Can you work these out from the model? Positions are in its coordinate system, mm. A direction names the side the tool comes from. Give positions to 0.01 mm unless a question says otherwise; leave off trailing zeros. Write each loop counter-clockwise with the first axis right and the second up, starting at its lowest first coordinate (ties: lowest second). Pieces come first, ordered by that corner, then holes.
from build123d import *

# Parameters (mm, degrees)
SKETCH1_R           = 10
BOSS_EXTRUDE1_DEPTH = 25
SKETCH2_R           = 4
CUT_EXTRUDE1_DEPTH  = 12.5
SKETCH3_R           = 2.5
CUT_EXTRUDE2_DEPTH  = 12.5
FILLET1_R           = 0.5
CHAMFER2_SIZE       = 0.5
CHAMFER3_SIZE       = 0.35
SKETCH4_R           = 3
CUT_EXTRUDE3_DEPTH  = 8
SKETCH5_R           = 1.25
CUT_EXTRUDE4_DEPTH  = 30.478806021
SKETCH6_W           = 1
SKETCH6_H           = 25
CUT_EXTRUDE5_DEPTH  = 13.95
SKETCH7_W           = 20.006481037
SKETCH7_H           = 0.5
CUT_EXTRUDE6_DEPTH  = 10.5
CUT_EXTRUDE7_START  = 13.975
SKETCH8_R           = 4
CUT_EXTRUDE7_DEPTH  = 13.975


with BuildPart() as part:
    # Sketch1 → Boss-Extrude1 (new body)
    with BuildSketch(Plane(origin=(0, 0, 0), x_dir=(1, 0, 0), z_dir=(0, 1, 0))):
        with Locations(Location((0, 0, 0), (0, 0, 270))):
            Circle(SKETCH1_R)
    extrude(amount=BOSS_EXTRUDE1_DEPTH)

    # Sketch2 → Cut-Extrude1 (cut)
    with BuildSketch(Plane(origin=(0, 25, 0), x_dir=(1, 0, 0), z_dir=(0, 1, 0))):
        with Locations(Location((0, 0, 0), (0, 0, 270))):
            Circle(SKETCH2_R)
    extrude(amount=-CUT_EXTRUDE1_DEPTH, mode=Mode.SUBTRACT)

    # Sketch3 → Cut-Extrude2 (cut)
    with BuildSketch(Plane.XZ):
        with Locations(Location((0, 0, 0), (0, 0, 270))):
            Circle(SKETCH3_R)
    extrude(amount=-CUT_EXTRUDE2_DEPTH, mode=Mode.SUBTRACT)

    # Fillet1
    fillet1_edges = [part.edges().sort_by_distance(p)[0] for p in [
        (0, 0, 2.5),
        (0, 25, -4),
    ]]
    fillet(fillet1_edges, radius=FILLET1_R)

    # Chamfer2
    chamfer2_edges = [part.edges().sort_by_distance(p)[0] for p in [
        (0, 12.5, 2.5),
    ]]
    chamfer(chamfer2_edges, length=CHAMFER2_SIZE)

    # Chamfer3
    chamfer3_edges = [part.edges().sort_by_distance(p)[0] for p in [
        (0, 0, -10),
        (0, 25, -10),
    ]]
    chamfer(chamfer3_edges, length=CHAMFER3_SIZE)

    # Sketch4 → Cut-Extrude3 (cut)
    with BuildSketch(Plane.ZY.offset(-10)):
        with Locations((-7, 19)):
            Circle(SKETCH4_R)
        with Locations((-7, 6)):
            Circle(SKETCH4_R)
    extrude(amount=CUT_EXTRUDE3_DEPTH, mode=Mode.SUBTRACT)

    # Sketch5 → Cut-Extrude4 (cut, through all)
    with BuildSketch(Plane(origin=(2, 0, 0), x_dir=(0, 0, -1), z_dir=(1, 0, 0))):
        with Locations((7, 19)):
            Circle(SKETCH5_R)
        with Locations((7, 6)):
            Circle(SKETCH5_R)
    extrude(amount=-CUT_EXTRUDE4_DEPTH, mode=Mode.SUBTRACT)

    # Sketch6 → Cut-Extrude5 (cut)
    with BuildSketch(Plane.XY.offset(-10)):
        with Locations((0, 12.5)):
            Rectangle(SKETCH6_W, SKETCH6_H)
    extrude(amount=CUT_EXTRUDE5_DEPTH, mode=Mode.SUBTRACT)

    # Sketch7 → Cut-Extrude6 (cut)
    with BuildSketch(Plane.ZY.offset(-10)):
        with Locations((0.003240519, 12.5)):
            Rectangle(SKETCH7_W, SKETCH7_H)
    extrude(amount=CUT_EXTRUDE6_DEPTH, mode=Mode.SUBTRACT)

    # Sketch8 → Cut-Extrude7 (cut)
    with BuildSketch(Plane(origin=(0, 12.25, 0), x_dir=(1, 0, 0), z_dir=(0, 1, 0)).offset(CUT_EXTRUDE7_START)):
        Circle(SKETCH8_R)
    extrude(amount=-CUT_EXTRUDE7_DEPTH, mode=Mode.SUBTRACT)


solid = part.part
(1) Imagine slicing it at D-D, the plane y = 6. Write out the boundary of the cut face in (x, z).
Returned:
outline: (-8.18, -5.75) - (-0.5, -5.75) - (-0.5, -2.45) arc R2.5 cw to (-0.5, 2.45) - (-0.5, 3.95) - (0.5, 3.95) - (0.5, 2.45) arc R2.5 cw to (0.5, -2.45) - (0.5, -5.75) - (2, -5.75) - (2, -4) - (9.17, -4) arc R10 ccw (long way) to start; (-5.65, -8.25) arc R10 ccw to (-0.5, -9.99) - (-0.5, -8.25) - close; (0.5, -9.99) arc R10 ccw to (2, -9.8) - (2, -8.25) - (0.5, -8.25) - close
(2) Imagine slicing it at B-B, the plane y = 19. Write out the boundary of the cut face in (x, z), plus the area to 3 significant figures.
Returned:
outline: (-8.18, -5.75) - (-0.5, -5.75) - (-0.5, -3.97) arc R4 cw (long way) to (0.5, -3.97) - (0.5, -5.75) - (2, -5.75) - (2, -4) - (9.17, -4) arc R10 ccw (long way) to start; (-5.65, -8.25) arc R10 ccw to (-0.5, -9.99) - (-0.5, -8.25) - close; (0.5, -9.99) arc R10 ccw to (2, -9.8) - (2, -8.25) - (0.5, -8.25) - close
area: 210 mm2
(3) If I drill on L1, parallel to Y at x = 0.9, z = -7; L2, parallel to Y at x = 6.5, z = 1.5; L3, parallel to Z at x = -2.5, y = 19, over which ranges is the centre line in solid material (lowest first)?
Returned:
L1: y = 0 to 4.75, 7.25 to 12.25, 12.75 to 17.75, 20.25 to 25
L2: y = 0 to 12.25, 12.75 to 25
L3: z = -9.68 to -8.25, -5.75 to -3.12, 3.12 to 9.68
(4) For faces 3 (the face through (-2.63, 12.13, 0.05)), 4 (the face through (0.5, 6, 3)), 5 (the face through (5, 6, -4)), which set-ups out of +Z, -Z, +X, -X, +Y, -Y let a thin tool reach every point of the face, with its end or its side?
Returned:
face 3: +Y
face 4: -Z, +Y, -Y
face 5: +X
(5) Imagine slicing it at A-A, the plane z = 0. Write out the boundary of the cut face in (x, y), plus the area to 3 significant figures.
Returned:
outline: (-10, 0.35) - (-9.65, 0) - (-3, 0) arc R0.5 ccw to (-2.5, 0.5) - (-2.5, 12) - (-2.75, 12.25) - (-4, 12.25) - (-4, 24.5) arc R0.5 ccw to (-4.5, 25) - (-9.65, 25) - (-10, 24.65) - close; (2.5, 0.5) arc R0.5 ccw to (3, 0) - (9.65, 0) - (10, 0.35) - (10, 12.25) - (2.75, 12.25) - (2.5, 12) - close; (4, 12.75) - (10, 12.75) - (10, 24.65) - (9.65, 25) - (4.5, 25) arc R0.5 ccw to (4, 24.5) - close
area: 333 mm2
(6) If we mould it in two halves opening along Z, with no side actions, what happens to faces 1 (the face through (2.3, 0, -2.3)), 2 (the face through (-3.43, 19.05, -5.75))? For each: +Z half, -Z half, draft (parallel to the pull), parting line (faces both ways), or undercut.
Returned:
face 1: draft
face 2: undercut
(7) Will these pins go through, and if not, where does the flat tip stop? P1, Ø4, axis at y = 5.5, z = -7.5, coming from the -X side; P2, Ø1.7, axis at y = 19, z = -7.5, coming from the +X side; P3, Ø0.8, axis at y = 7.5, z = 3.5, coming from the -X side.
Returned:
P1: stops at x = -8.35
P2: stops at x = 2
P3: stops at x = -9.51
(8) Imagine slicing it at C-C, the plane y = 10.75. Write out the boundary of the cut face in (x, z), plus the area to 3 significant figures.
Returned:
outline: (-0.5, -9.99) - (-0.5, -2.45) arc R2.5 cw to (-0.5, 2.45) - (-0.5, 3.95) - (0.5, 3.95) - (0.5, 2.45) arc R2.5 cw to (0.5, -2.45) - (0.5, -9.99) arc R10 ccw (long way) to start
area: 286 mm2
